```python
from build123d import *

# Parameters (mm, degrees)
SKETCH_1_W          = 44
SKETCH_1_H          = 16
EXTRUDE_1_DEPTH     = 90
SKETCH_2_W          = 55
SKETCH_2_H          = 5
CUT_EXTRUDE_1_DEPTH = 101.498756211
SKETCH_3_W          = 34
SKETCH_3_H          = 10
CUT_EXTRUDE_2_DEPTH = 95.021274188
SKETCH_4_W          = 44
SKETCH_4_H          = 67
EXTRUDE_2_DEPTH     = 24
SKETCH_5_W          = 30
SKETCH_5_H          = 17
CUT_EXTRUDE_3_DEPTH = 24
CUT_EXTRUDE_4_DEPTH = 106.166534601
SKETCH_7_R          = 15
CUT_EXTRUDE_5_DEPTH = 9
SKETCH_8_R          = 7.25
CUT_EXTRUDE_6_DEPTH = 98.698515854


with BuildPart() as part:
    # Эскиз1 → Бобышка-Вытянуть1 (new body)
    with BuildSketch(Plane.XY):
        Rectangle(SKETCH_1_W, SKETCH_1_H)
    extrude(amount=EXTRUDE_1_DEPTH)

    # Эскиз2 → Вырез-Вытянуть1 (cut, through all)
    with BuildSketch(Plane(origin=(22, 0, 0), x_dir=(0, 0, -1), z_dir=(1, 0, 0))):
        with Locations((-35.5, -5.5)):
            Rectangle(SKETCH_2_W, SKETCH_2_H)
    extrude(amount=-CUT_EXTRUDE_1_DEPTH, mode=Mode.SUBTRACT)

    # Эскиз3 → Вырез-Вытянуть2 (cut, through all)
    with BuildSketch(Plane(origin=(0, 8, 0), x_dir=(1, 0, 0), z_dir=(0, 1, 0))):
        with Locations((0, -85)):
            Rectangle(SKETCH_3_W, SKETCH_3_H)
    extrude(amount=-CUT_EXTRUDE_2_DEPTH, mode=Mode.SUBTRACT)

    # Эскиз4 → Бобышка-Вытянуть2 (add)
    with BuildSketch(Plane(origin=(0, 8, 0), x_dir=(1, 0, 0), z_dir=(0, 1, 0))):
        with Locations((0, -41.5)):
            Rectangle(SKETCH_4_W, SKETCH_4_H)
    extrude(amount=EXTRUDE_2_DEPTH)

    # Эскиз5 → Вырез-Вытянуть3 (cut)
    with BuildSketch(Plane(origin=(0, 32, 0), x_dir=(1, 0, 0), z_dir=(0, 1, 0))):
        with Locations((0, -66.5)):
            Rectangle(SKETCH_5_W, SKETCH_5_H)
    extrude(amount=-CUT_EXTRUDE_3_DEPTH, mode=Mode.SUBTRACT)

    # Эскиз6 → Вырез-Вытянуть4 (cut, through all)
    with BuildSketch(Plane(origin=(22, 0, 0), x_dir=(0, 0, -1), z_dir=(1, 0, 0))):
        Polygon((-75, 22), (-58, 32), (-75, 32), align=None)
    extrude(amount=-CUT_EXTRUDE_4_DEPTH, mode=Mode.SUBTRACT)

    # Эскиз7 → Вырез-Вытянуть5 (cut)
    with BuildSketch(Plane(origin=(0, 32, 0), x_dir=(1, 0, 0), z_dir=(0, 1, 0))):
        with Locations(Location((0, -33, 0), (0, 0, 270))):
            Circle(SKETCH_7_R)
    extrude(amount=-CUT_EXTRUDE_5_DEPTH, mode=Mode.SUBTRACT)

    # Эскиз8 → Вырез-Вытянуть6 (cut, through all)
    with BuildSketch(Plane(origin=(0, 23, 0), x_dir=(1, 0, 0), z_dir=(0, 1, 0))):
        with Locations(Location((0, -33, 0), (0, 0, 270))):
            Circle(SKETCH_8_R)
    extrude(amount=-CUT_EXTRUDE_6_DEPTH, mode=Mode.SUBTRACT)


solid = part.part
```
Could you check a few things on this model? Use its own coordinates, in mm. A direction names the side the tool comes from. Coordinates: 2 decimals unless noted, no trailing zeros. Write each loop counter-clockwise with the first axis right and the second up, starting at its lowest first coordinate (ties: lowest second). Pieces come first, ordered by that corner, then holes. Notation, with made-up numbers: (-24, 44.25) -> (31, 44.25) arc R21 ccw to (31, 53.25) -> close; hole circle Ø3 at (83.25, 66). An arc over 180 degrees is marked (long way). One line per question, with ' | ' between items. Start each with the question number.
1. For faces 1 (the face through (0, -3, 42)), 2 (the face through (17, 0, 85)), 3 (the face through (-19, 15, 75)), which set-ups out of +Z, -Z, +X, -X, +Y, -Y let a thin tool reach every point of the face, with its end or its side?
2. Please list where these lines run through material, in increasing order: line 1 along X through (y, z) = (13, 68); line 2 along X through (y, z) = (15, 33); line 3 along Y through (x, z) = (-14, 60).
3. Will these pins go through, and if not, where does the flat tip stop? P1, Ø6, axis at x = -6.5, z = 26.5, coming from the +Y side; P2, Ø2, axis at x = -4, y = 21, coming from the +Z side; P3, Ø18, axis at x = 0, z = 33, coming from the -Y side; P4, Ø8, axis at x = -2.5, z = 31.5, coming from the +Y side.
4. If we section it at B-B (y = 3.5): Please give me the cut outline in (x, z).
5. If we section it at D-D (y = 28): Please give me the cut outline in (x, z), and give its area (3 significant figures).
6. If we section it at A-A (z = 33): Please give me the cut outline in (x, y), and give its area (3 significant figures).
7. Thinking about a two-plate mould opening in Z: for faces 4 (the face through (0, -6, 8)), 5 (the face through (0, 20, 8)), 6 (the face through (19, 0, 90)), which applies, pulls with the +Z half, pulls with the -Z half, needs draft (parallel to the pull), parting line crosses it, or undercut?
8. If we section it at C-C (x = 3.5): Please give me the cut outline in (y, z), and give its area (3 significant figures).
Return value:
1) face 1: +X, -X, -Y | face 2: +Z, +Y, -Y | face 3: +Z, +X, -X, +Y
2) line 1: x = -22 to -15, 15 to 22 | line 2: x = -22 to -7.25, 7.25 to 22 | line 3: y = -3 to 8
3) P1: stops at y = 23 | P2: stops at z = 58 | P3: stops at y = -3 | P4: passes through
4) outline: (-22, 0) -> (22, 0) -> (22, 90) -> (17, 90) -> (17, 80) -> (-17, 80) -> (-17, 90) -> (-22, 90) -> close; hole circle Ø14.5 at (0, 33)
5) outline: (-22, 8) -> (22, 8) -> (22, 64.8) -> (15, 64.8) -> (15, 58) -> (-15, 58) -> (-15, 64.8) -> (-22, 64.8) -> close; hole circle Ø30 at (0, 33) | area: 1,590 mm²
6) outline: (-22, -3) -> (-7.25, -3) -> (-7.25, 23) -> (-15, 23) -> (-15, 32) -> (-22, 32) -> close; (7.25, -3) -> (22, -3) -> (22, 32) -> (15, 32) -> (15, 23) -> (7.25, 23) -> close | area: 893 mm²
7) face 4: undercut | face 5: pulls with the -Z half | face 6: pulls with the +Z half
8) outline: (-8, 0) -> (8, 0) -> (8, 8) -> (32, 8) -> (32, 18.41) -> (23, 18.41) -> (23, 26.65) -> (-3, 26.65) -> (-3, 8) -> (-8, 8) -> close; (-8, 63) -> (-3, 63) -> (-3, 39.35) -> (23, 39.35) -> (23, 47.59) -> (32, 47.59) -> (32, 58) -> (8, 58) -> (8, 80) -> (-8, 80) -> close | area: 1,610 mm²
